Geometry: see drawing. Coordinates: mm, zero at the bounding-box minimum. Round coordinates to 2 decimals unless told otherwise and drop trailing zeros. Loops run counter-clockwise (first coordinate to the right, second up) from the corner with the lowest first, then second, coordinate; pieces in that order, holes last.
(1) Material intervals for probe 1 along Y at (x, z) = (12, 15.5) (1 decimal); probe 2 along X at (y, z) = (9.5, 11) (1 decimal); probe 3 along X at (y, z) = (15.5, 5.5) (1 decimal), sorted ascending.
(2) Mould query, pull axis Y, two halves, no side actions, for the marked faces 1, 2 and 3. Classes: pulls with the +Y half, pulls with the -Y half, needs draft (parallel to the pull), parting line crosses it, or undercut.
(3) Section A-A, the plane z = 12.25. Return the cut outline in (x, y) (1 decimal).
(4) First-contact query: pin 1 Ø1 at (x, z) = (7.5, 9) entering from -Y; pin 2 Ø10 at (x, z) = (3, 4) entering from +Y; pin 3 Ø4 at (x, z) = (9, 2.5) entering from +Y; pin 4 Ø14 at (x, y) = (11.684, 11.684) entering from +Z. Flat tips, straight axial feed; report the tip coordinate or a pass-through.
(5) Section B-B, the plane z = 2. Return the cut outline in (x, y).
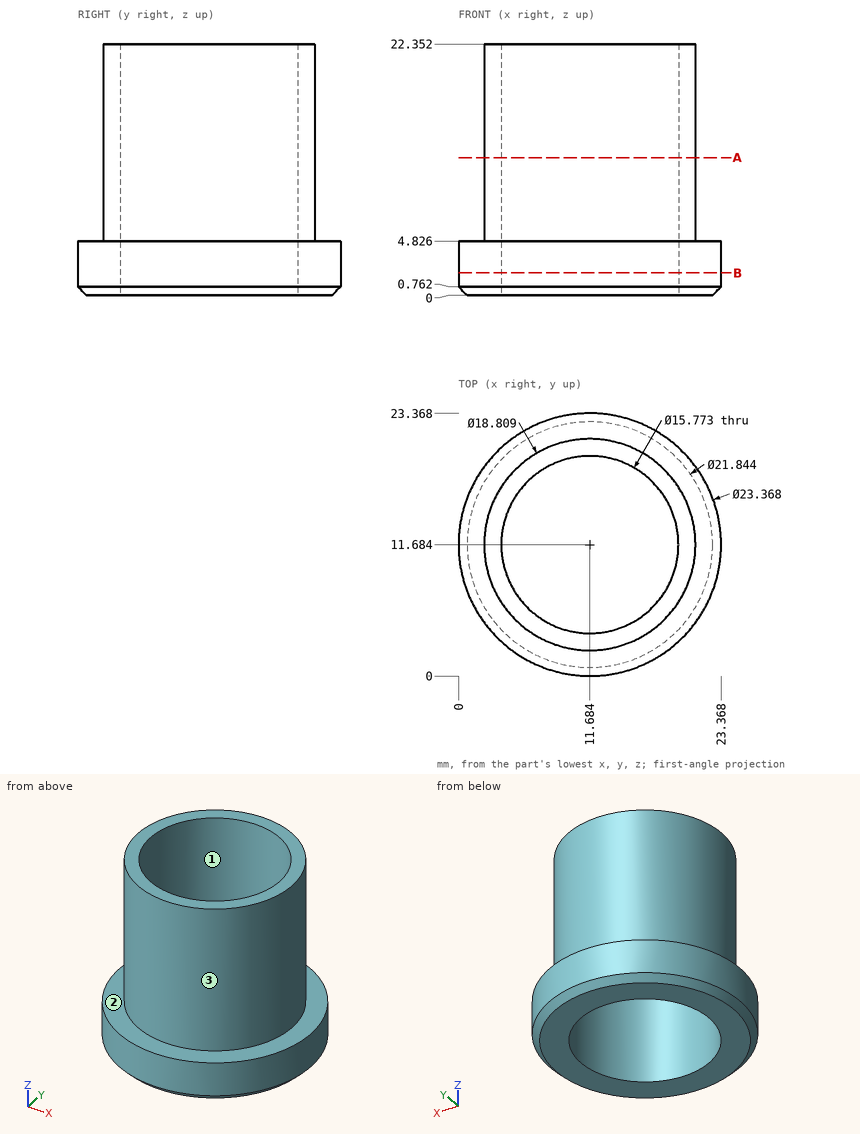
Output values:
1. probe 1: y = 2.3 to 3.8, 19.6 to 21.1
1. probe 2: x = 2.5 to 4.1, 19.3 to 20.8
1. probe 3: x = 3.1 to 4.8, 18.6 to 20.3
2. face 1: undercut
2. face 2: needs draft
2. face 3: parting line crosses it
3. outline: circle Ø18.8 at (11.7, 11.7); hole circle Ø15.8 at (11.7, 11.7)
4. pin 1: stops at y = 3.03
4. pin 2: stops at y = 22.77
4. pin 3: stops at y = 23.35
4. pin 4: passes through
5. outline: circle Ø23.37 at (11.68, 11.68); hole circle Ø15.77 at (11.68, 11.68)
